Geometry: final body of the model. Coordinates: model frame, mm. A direction names the side the tool comes from. Coordinates: 2 decimals unless noted, no trailing zeros. Write each loop counter-clockwise with the first axis right and the second up, starting at its lowest first coordinate (ties: lowest second). Pieces come first, ordered by that corner, then holes. Notation, with made-up numbers: (33, 36) - (80, 36) arc R21 cw to (80, 60) - close; hole circle Ø6 at (64.25, 49). An arc over 180 degrees is marked (long way). Answer as a JSON object with one key per item and string values. Group by question number.
Item 1: Mould query, pull axis X, two halves, no side actions, for faces 1 (the flat face through (51, 1, -100)), 2 (the cylindrical face through (4.05, 2.51, -4.12)), 3 (the flat face through (100, 1, -49)). Classes: pulls with the +X half, pulls with the -X half, needs draft (parallel to the pull), parting line crosses it, or undercut.
Item 2: Section A-A on z = -25.5. Return loops of the section in (x, y), and give its area (3 significant figures).
Item 3: Line query: line 1 along X through (y, z) = (2.4, -5.5); line 2 along Z through (x, y) = (5.5, 2.5); line 3 along Z through (x, y) = (61, 2.4). Output: solid intervals per line, ascending. Write a range as from..to.
Item 4: Set-up query: faces 4 (the flat face through (51, 0, -49)), 5 (the cylindrical face through (83.98, 2.51, -4.05)). Return all of +Z, -Z, +X, -X, +Y, -Y with unobstructed straight access to the full face (end or side cutting, diameter ignored); none if empty.
Item 5: First-contact query: pin 1 Ø4 at (x, z) = (55, -74) entering from +Y. Flat tip, straight axial feed; report the tip coordinate or a pass-through.
Item 6: Section B-B on x = 36. Return loops of the section in (y, z).
Autodesk Inventor part; units mm, degrees
ref_plane "YZ Plane" through (0, 0, 0) normal (1, 0, 0) x (0, 1, 0)
ref_plane "XZ Plane" through (0, 0, 0) normal (0, 1, 0) x (-1, 0, 0)
ref_plane "XY Plane" through (0, 0, 0) normal (0, 0, 1) x (1, 0, 0)
sketch "Sketch1" plane through (0, 0, 0) normal (0, 1, 0) x (-1, 0, 0)
  line L0 (0, 0) -> (-100, 0)
  line L1 (-100, 0) -> (-100, -100)
  line L2 (-100, -100) -> (0, -100)
  line L3 (0, -100) -> (0, 0)
  dimension "d0" = 100
  dimension "d1" = 100
extrude "Extrusion1" add sketch "Sketch1" along normal blind 3
sketch "Sketch2" plane through (0, 3, 0) normal (0, 1, 0) x (1, 0, 0)
  line L0 (5, 5) -> (83.1, 5)
  line L1 (83.1, 5) -> (83.1, 77.1)
  line L2 (83.1, 77.1) -> (5, 77.1)
  line L3 (5, 77.1) -> (5, 5)
  line L4 (0, 0) -> (100, 0)
  line L5 (0, 100) -> (0, 0)
  arc A0 (5, 7.4365) -> (7.4365, 5) centre (5.5, 5.5) ccw
  line L6 (44.05, 77.1) -> (44.05, 5) construction
  line L7 (5, 41.05) -> (83.1, 41.05) construction
  arc A1 (80.6635, 5) -> (83.1, 7.4365) centre (82.6, 5.5) ccw
  arc A2 (7.4365, 77.1) -> (5, 74.6635) centre (5.5, 76.6) ccw
  arc A3 (83.1, 74.6635) -> (80.6635, 77.1) centre (82.6, 76.6) ccw
  point P0 (80.6635, 5)
  point P1 (83.1, 7.4365)
  point P2 (83.1, 74.6635)
  point P3 (80.6635, 77.1)
  point P4 (7.4365, 77.1)
  point P5 (5, 74.6635)
  dimension "d4" = 78.1
  dimension "d5" = 72.1
  dimension "d6" = 5
  dimension "d7" = 5
  dimension "d10" = 0.5
  dimension "d11" = 0.5
  dimension "d12" = 2
extrude "Extrusion2" cut sketch "Sketch2" against normal blind 1
fillet "Fillet1" radius 1 8 edges at (5, 2.5, -7.4365) (7.4365, 2.5, -5) (83.1, 2.5, -7.4365) (80.6635, 2.5, -5) (83.1, 2.5, -74.6635) (80.6635, 2.5, -77.1) (7.4365, 2.5, -77.1) (5, 2.5, -74.6635)
Checks:
{
 "1": {"face 1": "needs draft", "face 2": "undercut", "face 3": "pulls with the +X half"},
 "2": {"outline": "(0, 0) - (100, 0) - (100, 3) - (83.1, 3) - (83.1, 2) - (5, 2) - (5, 3) - (0, 3) - close", "area": "222 mm^2"},
 "3": {"line 1": "0..3.5, 84.6..100", "line 2": "-100..-78.6, -3.5..0", "line 3": "-100..-77.1, -5..0"},
 "4": {"face 4": "+Z, -Z, +X, -X, -Y", "face 5": "+Y"},
 "5": {"pin 1": "y = 2"},
 "6": {"outline": "(0, -100) - (3, -100) - (3, -77.1) - (2, -77.1) - (2, -5) - (3, -5) - (3, 0) - (0, 0) - close"}
}
